Geometry: final body of the model. Coordinates: model frame, mm. A direction names the side the tool comes from. Round coordinates to 2 decimals unless told otherwise and drop trailing zeros. Loops run counter-clockwise (first coordinate to the right, second up) from the corner with the lowest first, then second, coordinate; pieces in that order, holes last. Notation, with made-up numbers: (56, 67.5) -> (113, 67.5) arc R31 cw to (113, 91.5) -> close; hole circle Ø9 at (-9.75, 68). An arc over 180 degrees is marked (long way). Answer in a Markdown table with one row per item.
```python
from build123d import *

# Parameters (mm, degrees)
SKETCH1_R           = 10
BOSS_EXTRUDE1_DEPTH = 20
SKETCH2_R           = 25
BOSS_EXTRUDE2_DEPTH = 22
SKETCH3_R           = 20.5
CUT_EXTRUDE1_DEPTH  = 20
FILLET1_R           = 5
SKETCH4_R           = 7.35
CUT_EXTRUDE2_DEPTH  = 20
SKETCH5_R           = 8.25
BOSS_EXTRUDE3_DEPTH = 37.5
SKETCH6_R           = 4.5
CUT_EXTRUDE3_DEPTH  = 30
SKETCH7_R           = 25
SKETCH7_R_2         = 20.5
CUT_EXTRUDE4_DEPTH  = 8


with BuildPart() as part:
    # Sketch1 → Boss-Extrude1 (new body)
    with BuildSketch(Plane(origin=(0, 0, 0), x_dir=(1, 0, 0), z_dir=(0, 1, 0))):
        with Locations(Location((0, 0, 0), (0, 0, 270))):
            Circle(SKETCH1_R)
    extrude(amount=BOSS_EXTRUDE1_DEPTH)

    # Sketch2 → Boss-Extrude2 (add)
    with BuildSketch(Plane.XZ):
        with Locations(Location((0, 0, 0), (0, 0, 270))):
            Circle(SKETCH2_R)
    extrude(amount=BOSS_EXTRUDE2_DEPTH)

    # Sketch3 → Cut-Extrude1 (cut)
    with BuildSketch(Plane.XZ.offset(22)):
        with Locations(Location((0, 0, 0), (0, 0, 270))):
            Circle(SKETCH3_R)
    extrude(amount=-CUT_EXTRUDE1_DEPTH, mode=Mode.SUBTRACT)

    # Fillet1
    fillet1_edges = [part.edges().sort_by_distance(p)[0] for p in [
        (0, 0, 25),
    ]]
    fillet(fillet1_edges, radius=FILLET1_R)

    # Sketch4 → Cut-Extrude2 (cut)
    with BuildSketch(Plane(origin=(0, 20, 0), x_dir=(1, 0, 0), z_dir=(0, 1, 0))):
        with Locations(Location((0, 0, 0), (0, 0, 270))):
            Circle(SKETCH4_R)
    extrude(amount=-CUT_EXTRUDE2_DEPTH, mode=Mode.SUBTRACT)

    # Sketch5 → Boss-Extrude3 (add)
    with BuildSketch(Plane.XZ.offset(2)):
        with Locations(Location((0, 11.748259103, 0), (0, 0, 270))):
            Circle(SKETCH5_R)
        with Locations(Location((0, -11.748259103, 0), (0, 0, 270))):
            Circle(SKETCH5_R)
    extrude(amount=BOSS_EXTRUDE3_DEPTH)

    # Sketch6 → Cut-Extrude3 (cut)
    with BuildSketch(Plane.XZ.offset(39.5)):
        with Locations(Location((0, 11.748259103, 0), (0, 0, 270))):
            Circle(SKETCH6_R)
        with Locations(Location((0, -11.748259103, 0), (0, 0, 270))):
            Circle(SKETCH6_R)
    extrude(amount=-CUT_EXTRUDE3_DEPTH, mode=Mode.SUBTRACT)

    # Sketch7 → Cut-Extrude4 (cut)
    with BuildSketch(Plane.XZ.offset(22)):
        with Locations(Location((0, 0, 0), (0, 0, 270))):
            Circle(SKETCH7_R)
        with Locations(Location((0, 0, 0), (0, 0, 270))):
            Circle(SKETCH7_R_2, mode=Mode.SUBTRACT)
    extrude(amount=-CUT_EXTRUDE4_DEPTH, mode=Mode.SUBTRACT)


solid = part.part
```
Item 1: Ray query, L1, parallel to X at y = 15, z = 0; L2, parallel to X at y = -11, z = 6.5; L3, parallel to X at y = -12.5, z = 0. Return the intervals inside material, ascending.
Ans:
| item | result |
|---|---|
| L1 | -10 to -7.35, 7.35 to 10 |
| L2 | -24.14 to -19.44, -6.37 to 6.37, 19.44 to 24.14 |
| L3 | -25 to -20.5, 20.5 to 25 |
Item 2: Section query A-A, the plane z = 0. Output: boundary loops of the cut face in (x, y).
Ans:
| item | result |
|---|---|
| outline | (-25, -14) -> (-20.5, -14) -> (-20.5, -2) -> (20.5, -2) -> (20.5, -14) -> (25, -14) -> (25, -5) arc R5 ccw to (20, 0) -> (10, 0) -> (10, 20) -> (7.35, 20) -> (7.35, 0) -> (-7.35, 0) -> (-7.35, 20) -> (-10, 20) -> (-10, 0) -> (-20, 0) arc R5 ccw to (-25, -5) -> close |
Item 3: Set-up query: faces 5 (the flat face through (7.5, 20, 0)), 6 (the flat face through (0, -2, 0)), 7 (the flat face through (9, 0, 5)). Return all of +Z, -Z, +X, -X, +Y, -Y with unobstructed straight access to the full face (end or side cutting, diameter ignored); none if empty.
Ans:
| item | result |
|---|---|
| face 5 | +Z, -Z, +X, -X, +Y |
| face 6 | -Y |
| face 7 | +Y |
Item 4: Section query B-B, the plane y = -21.5. Output: boundary loops of the cut face in (x, z).
Ans:
| item | result |
|---|---|
| outline | circle Ø16.5 at (0, -11.75); circle Ø16.5 at (0, 11.75); hole circle Ø9 at (0, -11.75); hole circle Ø9 at (0, 11.75) |
Item 5: First-contact query: P1, Ø5, axis at x = -17.5, y = -0.5, coming from the +Z side; P2, Ø3, axis at y = -18.5, z = 13, coming from the +X side; P3, Ø8, axis at x = -19.5, y = -4.5, coming from the +Z side. Flat tips, straight axial feed; report the tip coordinate or a pass-through.
Ans:
| item | result |
|---|---|
| P1 | z = 18.37 |
| P2 | x = 8.25 |
| P3 | z = 19.6 |
Item 6: Mould query, pull axis X, two halves, no side actions, for faces 1 (the cylindrical face through (0.198, -24.71, -7.253)), 2 (the flat face through (0, -9.5, -12)), 3 (the cylindrical face through (-9.76, 9.86, -2.17)), 4 (the flat face through (-4, -39.5, -15)). Classes: released by +X, released by -X, zero draft, split by the parting line, or undercut.
Ans:
| item | result |
|---|---|
| face 1 | undercut |
| face 2 | undercut |
| face 3 | split by the parting line |
| face 4 | zero draft |
